Study the drawing (mm; zero at the part's minimum x, y, z) and answer. A direction names the side the tool comes from. Round coordinates to 2 decimals unless told otherwise and drop trailing zeros. Write each loop counter-clockwise with the first axis right and the second up, starting at its lowest first coordinate (ties: lowest second). Pieces come first, ordered by that corner, then holes.
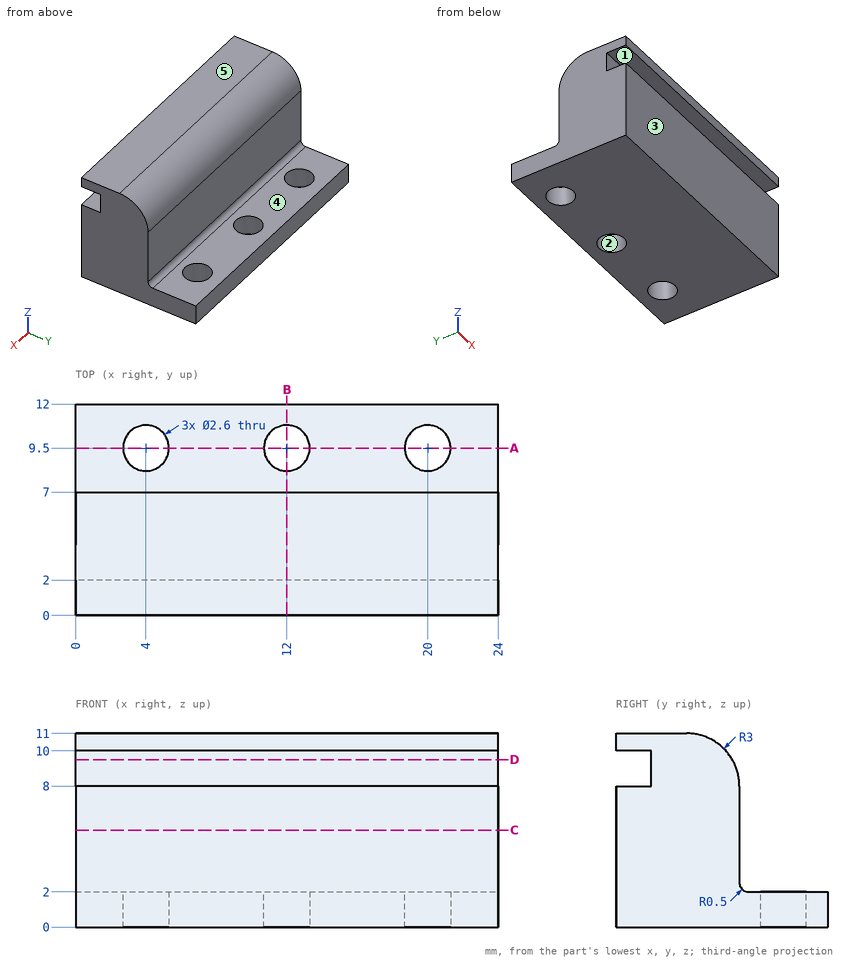
1. Given pin 1 (6 mm diameter, centred on y = 7.5, z = 3, fed in from -X); pin 2 (5 mm diameter, centred on x = 13, y = 10, fed in from +Z); pin 3 (2.5 mm diameter, centred on x = 20, y = 9.5, fed in from -Z); pin 4 (4.5 mm diameter, centred on x = 9.5, z = 4.5, fed in from +Y), each flat-ended and moving along its own axis, determine where each tip first touches the part or whether it passes through.
Geometry says:
pin 1: stops at x = 0
pin 2: stops at z = 2
pin 3: passes through
pin 4: stops at y = 7.07
2. Straight lines are drawn through the part: line 1 along Z through (x, y) = (13.5, 1); line 2 along Y through (x, z) = (4, 1.55); line 3 along Y through (x, z) = (16.5, 4.25). For each, find the intervals that lie inside material, in ascending order.
Geometry says:
line 1: z = 0 to 8, 10 to 11
line 2: y = 0 to 8.2, 10.8 to 12
line 3: y = 0 to 7
3. Section D-D on z = 9.5 is taken. Determine the outline of the cut face in (x, y).
Geometry says:
outline: (0, 2) - (24, 2) - (24, 6.6) - (0, 6.6) - close
4. Section A-A on y = 9.5 is taken. Determine the outline of the cut face in (x, z).
Geometry says:
outline: (0, 0) - (2.7, 0) - (2.7, 2) - (0, 2) - close; (5.3, 0) - (10.7, 0) - (10.7, 2) - (5.3, 2) - close; (13.3, 0) - (18.7, 0) - (18.7, 2) - (13.3, 2) - close; (21.3, 0) - (24, 0) - (24, 2) - (21.3, 2) - close
5. Section C-C on z = 5.5 is taken. Determine the outline of the cut face in (x, y).
Geometry says:
outline: (0, 0) - (24, 0) - (24, 7) - (0, 7) - close
6. For a pull along Y with two mould halves and no side action, classify the marked faces 1, 2 and 3 as released by +Y, released by -Y, zero draft, split by the parting line, or undercut.
Geometry says:
face 1: zero draft
face 2: undercut
face 3: released by -Y
7. A tool of negligible diameter and unlimited length cuts with its end or side. For the marked faces 4 and 5, from which of +Z, -Z, +X, -X, +Y, -Y can it reach the whole face along a straight path? Write none if from no direction.
Geometry says:
face 4: +Z, +X, -X, +Y
face 5: +Z, +X, -X, +Y, -Y
8. Section B-B on x = 12 is taken. Determine the outline of the cut face in (y, z).
Geometry says:
outline: (0, 0) - (8.2, 0) - (8.2, 2) - (7.5, 2) arc R0.5 cw to (7, 2.5) - (7, 8) arc R3 ccw to (4, 11) - (0, 11) - (0, 10) - (2, 10) - (2, 8) - (0, 8) - close; (10.8, 0) - (12, 0) - (12, 2) - (10.8, 2) - close
